Source: CAD feature listing. Evaluate the final solid. Frame: model axes, mm. Coordinates: 2 decimals unless noted, no trailing zeros. Order: outer loops, then holes, each group sorted by start corner. A loop starts at its lowest first (then second) coordinate and runs counter-clockwise, first axis right, second up. Notation, with made-up numbers: (76.25, -2.5) -> (81.25, -2.5) arc R15 cw to (81.25, 18.5) -> close; hole circle Ø11 at (-20.75, -5). An arc over 180 degrees is marked (long way). Write item = value, one per line. Start each with the question number.
Item 1: Contact query for a flat-ended pin moving along its axis: pin 1 (2 mm diameter, centred on x = -86.5, y = 128, fed in from -Z). Output: stop coordinate, or through.
Item 2: Section query C-C (z = 0.5). Output: boundary loops of the cut face in (x, y) (1 decimal).
Item 3: Ray query, line 1 along Y through (x, z) = (-38.1, 0.9); line 2 along X through (y, z) = (128, 0.8); line 3 along Y through (x, z) = (-42, 1.1). Return the intervals inside material, ascending. Write a range as [from, to].
Item 4: Section query A-A (y = 127). Output: boundary loops of the cut face in (x, z).
Item 5: Mould query, pull axis X, two halves, no side actions, for faces 1 (the flat face through (-39, 142, 0)), 2 (the cylindrical face through (-32.63, 140.2, 0.8)). Classes: released by +X, released by -X, zero draft, split by the parting line, or undercut.
Item 6: Section query B-B (x = -31.5). Output: boundary loops of the cut face in (y, z), then the cut area to 3 significant figures.
Autodesk Inventor part; units mm, degrees
ref_plane "YZ Plane" through (0, 0, 0) normal (1, 0, 0) x (0, 1, 0)
ref_plane "XZ Plane" through (0, 0, 0) normal (0, 1, 0) x (-1, 0, 0)
ref_plane "XY Plane" through (0, 0, 0) normal (0, 0, 1) x (1, 0, 0)
sketch "Sketch1" plane through (0, 0, 0) normal (0, 0, 1) x (1, 0, 0)
  line L0 (25.4, 63.5) -> (-101.6, 63.5)
  line L1 (-101.6, 63.5) -> (-101.6, 190.5)
  line L2 (-101.6, 190.5) -> (25.4, 190.5)
  line L3 (25.4, 190.5) -> (25.4, 63.5)
  point P0 (0, 0)
  dimension "d0" = 127
  dimension "d1" = 127
extrude "Extrusion1" add sketch "Sketch1" along normal blind 1.5875
sketch "Sketch2" plane through (0, 0, 0) normal (0, 0, -1) x (-1, 0, 0)
  line L0 (-25.4, 63.5) -> (101.6, 63.5)
  line L1 (101.6, 63.5) -> (101.6, 190.5)
  line L2 (101.6, 190.5) -> (-25.4, 190.5)
  line L3 (-25.4, 190.5) -> (-25.4, 63.5)
  line L4 (38.1, 190.5) -> (38.1, 127)
  point P0 (0, 0)
  dimension "d4" = 127
  dimension "d5" = 127
  dimension "d6" = 63.5
hole "Hole1" at (-38.1, 127, 0) direction (0, 0, 1) diameter 28.575 end through all
properties part number "mountingPanelCannon"
Computed:
q1.pin_1 = 0
q2.outline = (-101.6, 63.5) -> (25.4, 63.5) -> (25.4, 190.5) -> (-101.6, 190.5) -> close; hole circle Ø28.6 at (-38.1, 127)
q3.line_1 = [63.5, 112.71], [141.29, 190.5]
q3.line_2 = [-101.6, -52.35], [-23.85, 25.4]
q3.line_3 = [63.5, 113.26], [140.74, 190.5]
q4.outline = (-101.6, 0) -> (-52.39, 0) -> (-52.39, 1.59) -> (-101.6, 1.59) -> close; (-23.81, 0) -> (25.4, 0) -> (25.4, 1.59) -> (-23.81, 1.59) -> close
q5.face_1 = zero draft
q5.face_2 = undercut
q6.outline = (63.5, 0) -> (114.33, 0) -> (114.33, 1.59) -> (63.5, 1.59) -> close; (139.67, 0) -> (190.5, 0) -> (190.5, 1.59) -> (139.67, 1.59) -> close
q6.area = 161 mm^2
